Could you check a few things on this model? Use its own coordinates, in mm. Face numbers are marked on the shaded views. A direction names the side the tool comes from. Round coordinates to 2 decimals unless told otherwise and drop trailing zeros. Order: outer loops, then holes, each group sorted by start corner. A loop starts at its lowest first (then second) coordinate and runs counter-clockwise, first axis right, second up. Notation, with made-up numbers: (86.25, 85) -> (112.25, 85) arc R13 cw to (112.25, 99) -> close; hole circle Ø6 at (6.25, 69). An arc over 180 degrees is marked (long way). Put each result on its own line as item: value. Start each with the question number.
from build123d import *

# Parameters (mm, degrees)
ESTRUSIONE_ESTRUSIONE1_DEPTH                         = 23
FORO_PER_VITE_M4_1_D                                 = 5.6
FORO_PER_VITE_M4_1_DEPTH                             = 10
FORO_PER_VITE_M4_1_TIP                               = 1.682409733
FORO_LAMATO_PER_BULLONE_M5_A_TESTA_ESAGO_D           = 4.5
FORO_LAMATO_PER_BULLONE_M5_A_TESTA_ESAGO_DEPTH       = 10
FORO_LAMATO_PER_BULLONE_M5_A_TESTA_ESAGO_CBORE_D     = 10
FORO_LAMATO_PER_BULLONE_M5_A_TESTA_ESAGO_CBORE_DEPTH = 3
FORO_LAMATO_PER_BULLONE_M5_A_TESTA_ESAGO_TIP         = 1.351936393


with BuildPart() as part:
    # Schizzo1 → Estrusione-Estrusione1 (new body)
    with BuildSketch(Plane.XY):
        Polygon((0, 0), (20, 0), (20, 12), (40, 12), (40, 16), (20, 16), (7, 12), (0, 12), align=None)
    extrude(amount=ESTRUSIONE_ESTRUSIONE1_DEPTH)

    # Foro per Vite M4-1
    with Locations(Plane(origin=(0, 5.5, 5), x_dir=(0, -1, 0), z_dir=(-1, 0, 0))):
        with Locations((0, 0), (0, 13)):
            Hole(FORO_PER_VITE_M4_1_D / 2, depth=FORO_PER_VITE_M4_1_DEPTH)
            with Locations((0, 0, -(FORO_PER_VITE_M4_1_DEPTH + FORO_PER_VITE_M4_1_TIP / 2))):  # 118° drill point
                Cone(0, FORO_PER_VITE_M4_1_D / 2, FORO_PER_VITE_M4_1_TIP, mode=Mode.SUBTRACT)

    # Foro lamato per Bullone M5 a testa esagonale-1
    with Locations(Plane(origin=(0, 16, 0), x_dir=(1, 0, 0), z_dir=(0, 1, 0))):
        with Locations((30, -11.5)):
            CounterBoreHole(FORO_LAMATO_PER_BULLONE_M5_A_TESTA_ESAGO_D / 2, FORO_LAMATO_PER_BULLONE_M5_A_TESTA_ESAGO_CBORE_D / 2, FORO_LAMATO_PER_BULLONE_M5_A_TESTA_ESAGO_CBORE_DEPTH, depth=FORO_LAMATO_PER_BULLONE_M5_A_TESTA_ESAGO_DEPTH)
            with Locations((0, 0, -(FORO_LAMATO_PER_BULLONE_M5_A_TESTA_ESAGO_DEPTH + FORO_LAMATO_PER_BULLONE_M5_A_TESTA_ESAGO_TIP / 2))):  # 118° drill point
                Cone(0, FORO_LAMATO_PER_BULLONE_M5_A_TESTA_ESAGO_D / 2, FORO_LAMATO_PER_BULLONE_M5_A_TESTA_ESAGO_TIP, mode=Mode.SUBTRACT)


solid = part.part
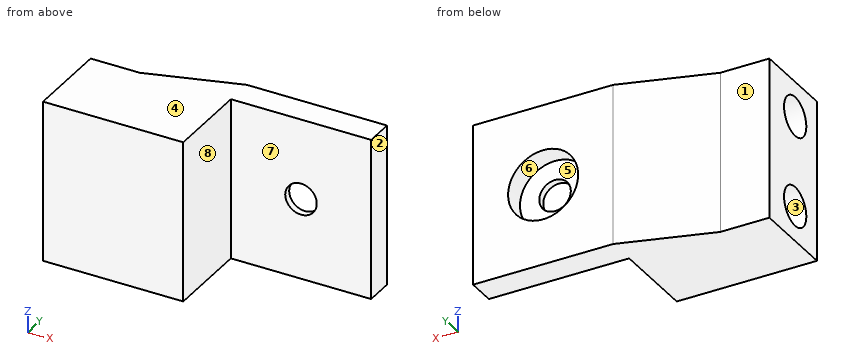
1. For pin 1 Ø7.5 at (y, z) = (5.5, 18) entering from +X; pin 2 Ø2 at (x, z) = (3, 13.5) entering from +Y; pin 3 Ø5 at (x, z) = (30, 11.5) entering from +Y, each with a flat end and sliding along its axis, tell me the tip position at first contact or that it passes through.
2. If we section it at A-A, the plane z = 11.5: Please give me the cut outline in (x, y), then the cut area to 4 significant figures.
3. If we section it at D-D, the plane y = 9: Please give me the cut outline in (x, z).
4. Which directions (+Z, -Z, +X, -X, +Y, -Y) give clear straight access to the entire face, cutting with the end or side of a thin tool? Please do the marked faces 1, 2, 3, 4 and 5.
5. If we section it at C-C, the plane y = 14: Please give me the cut outline in (x, z).
6. Thinking about a two-plate mould opening in X: for the marked faces 6, 7 and 8, which applies, +X half, -X half, draft (parallel to the pull), parting line (faces both ways), or undercut?
7. If we section it at B-B, the plane x = 26: Please give me the cut outline in (y, z), then the cut area to 3 significant figures.
8. I need wall thicknesses on L1, parallel to Z at x = 6.25, y = 5.5; L2, parallel to Z at x = 30, y = 12.4; L3, parallel to Y at x = 3.25, z = 5. Which ranges of each line are inside material? Lowest first, please.
Results below:
1. pin 1: x = 20
1. pin 2: y = 12
1. pin 3: y = 13
2. outline: (0, 0) -> (20, 0) -> (20, 12) -> (27.75, 12) -> (27.75, 13) -> (25, 13) -> (25, 16) -> (20, 16) -> (7, 12) -> (0, 12) -> close; (32.25, 12) -> (40, 12) -> (40, 16) -> (35, 16) -> (35, 13) -> (32.25, 13) -> close
2. area: 311.5 mm2
3. outline: (0, 0) -> (20, 0) -> (20, 23) -> (0, 23) -> close
4. face 1: +Z, -Z, -X, +Y
4. face 2: +Z, -Z, +X, +Y, -Y
4. face 3: -X
4. face 4: +Z, +X, -X, +Y, -Y
4. face 5: +Y
5. outline: (13.5, 0) -> (40, 0) -> (40, 23) -> (13.5, 23) -> close; hole circle Ø10 at (30, 11.5)
6. face 6: undercut
6. face 7: draft
6. face 8: +X half
7. outline: (12, 0) -> (16, 0) -> (16, 8.5) -> (13, 8.5) -> (13, 14.5) -> (16, 14.5) -> (16, 23) -> (12, 23) -> close
7. area: 74.0 mm2
8. L1: 0 to 2.2, 7.8 to 15.2, 20.8 to 23
8. L2: 0 to 9.25, 13.75 to 23
8. L3: 0 to 2.7, 8.3 to 12
